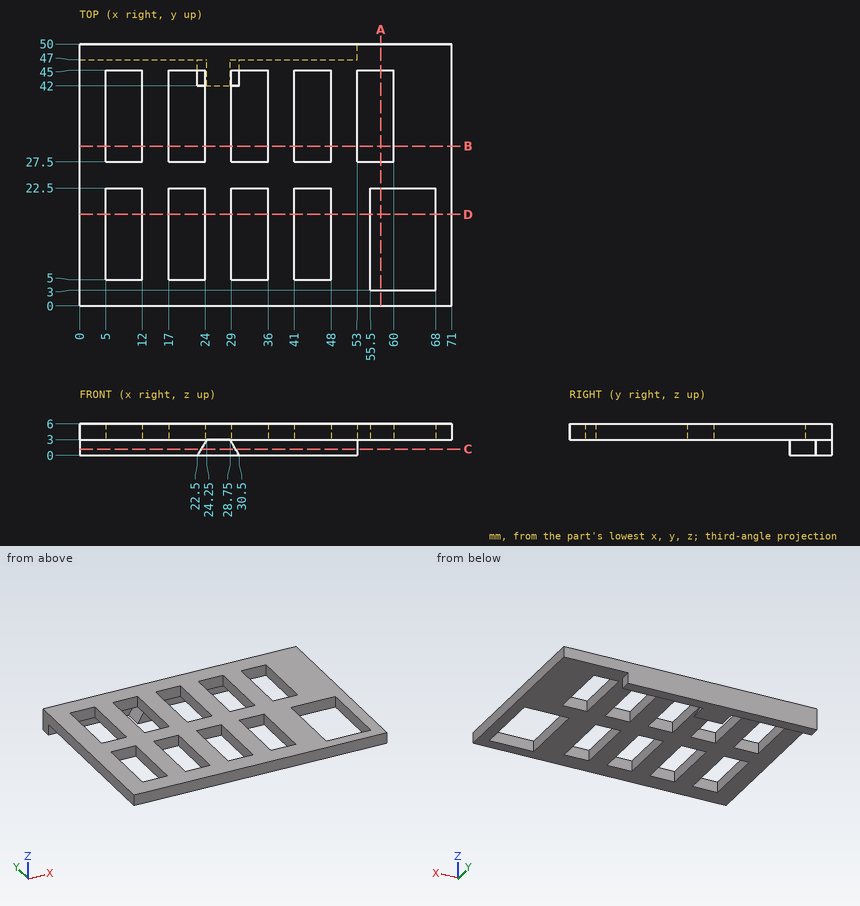
Could you check a few things on this drawing? It's one solid part, dimensions in mm from its lowest x, y, z. Round coordinates to 2 decimals unless told otherwise and drop trailing zeros. Write each loop counter-clockwise with the first axis right and the second up, starting at its lowest first coordinate (ties: lowest second). Pieces come first, ordered by that corner, then holes. Notation, with made-up numbers: (31.5, -25.5) -> (56.5, -25.5) arc R30 ccw to (56.5, 0.5) -> close; hole circle Ø6 at (25, 38). An arc over 180 degrees is marked (long way). Use a Markdown table: item, result.
1. For pin 1 Ø0.9 at (x, z) = (36.5, 1) entering from -Y, with a flat end and sliding along its axis, tell me the tip position at first contact or that it passes through.
Answer key:
| item | result |
|---|---|
| pin 1 | stops at y = 47 |
2. If we section it at C-C (z = 1.2): List the corners of the cut face in (x, y) for me, then the cut area to 3 significant figures.
Answer key:
| item | result |
|---|---|
| outline | (0, 47) -> (23.2, 47) -> (23.2, 42) -> (29.8, 42) -> (29.8, 47) -> (53, 47) -> (53, 50) -> (0, 50) -> close |
| area | 192 mm^2 |
3. If we section it at B-B (y = 30.5): List the corners of the cut face in (x, z) for me, then the cut area to 3 significant figures.
Answer key:
| item | result |
|---|---|
| outline | (0, 3) -> (5, 3) -> (5, 6) -> (0, 6) -> close; (12, 3) -> (17, 3) -> (17, 6) -> (12, 6) -> close; (24, 3) -> (29, 3) -> (29, 6) -> (24, 6) -> close; (36, 3) -> (41, 3) -> (41, 6) -> (36, 6) -> close; (48, 3) -> (53, 3) -> (53, 6) -> (48, 6) -> close; (60, 3) -> (71, 3) -> (71, 6) -> (60, 6) -> close |
| area | 108 mm^2 |
4. If we section it at A-A (x = 57.5): List the corners of the cut face in (y, z) for me.
Answer key:
| item | result |
|---|---|
| outline | (0, 3) -> (3, 3) -> (3, 6) -> (0, 6) -> close; (22.5, 3) -> (27.5, 3) -> (27.5, 6) -> (22.5, 6) -> close; (45, 3) -> (50, 3) -> (50, 6) -> (45, 6) -> close |
5. Please list where these lines run through material, in increasing order: probe 1 along X at (y, z) = (33, 4.9); probe 2 along Y at (x, z) = (7.5, 5.7); probe 3 along Y at (x, z) = (57, 5.6).
Answer key:
| item | result |
|---|---|
| probe 1 | x = 0 to 5, 12 to 17, 24 to 29, 36 to 41, 48 to 53, 60 to 71 |
| probe 2 | y = 0 to 5, 22.5 to 27.5, 45 to 50 |
| probe 3 | y = 0 to 3, 22.5 to 27.5, 45 to 50 |
6. If we section it at D-D (y = 17.5): List the corners of the cut face in (x, z) for me, then the cut area to 3 significant figures.
Answer key:
| item | result |
|---|---|
| outline | (0, 3) -> (5, 3) -> (5, 6) -> (0, 6) -> close; (12, 3) -> (17, 3) -> (17, 6) -> (12, 6) -> close; (24, 3) -> (29, 3) -> (29, 6) -> (24, 6) -> close; (36, 3) -> (41, 3) -> (41, 6) -> (36, 6) -> close; (48, 3) -> (55.5, 3) -> (55.5, 6) -> (48, 6) -> close; (68, 3) -> (71, 3) -> (71, 6) -> (68, 6) -> close |
| area | 91.5 mm^2 |
